Could you check a few things on this model? Use its own coordinates, in mm. Face numbers are marked on the shaded views. A direction names the side the tool comes from. Round coordinates to 2 decimals unless told otherwise and drop trailing zeros. Order: outer loops, then holes, each group sorted by start corner. A loop starts at its lowest first (then second) coordinate and runs counter-clockwise, first axis right, second up. Notation, with made-up numbers: M 75.5,-36.75 L 101.5,-36.75 A31 cw 101.5,-10.75 Z; hole C 25,53 d9. An arc over 180 degrees is marked long. Write each question's results on one line, items separated by ' | '. Start each with the question number.
1. Suppose I cut it at C-C on x = -107. Write out the boundary of the cut face in (y, z), and give its area (3 significant figures).
2. Suppose I cut it at A-A on y = 0. Write out the boundary of the cut face in (x, z), and give its area (3 significant figures).
3. I'm going to push flat-ended pins straight in: pin 1 (1.5 mm diameter, centred on x = -146.5, z = 86, fed in from -Y) (3 decimals); pin 2 (8 mm diameter, centred on y = 8.5, z = 84, fed in from +X); pin 3 (10 mm diameter, centred on y = -5, z = 49.5, fed in from +X). Where does each tip first touch, or does it pass through?
4. For the marked faces 1 and 2, which set-ups out of +Z, -Z, +X, -X, +Y, -Y let a thin tool reach every point of the face, with its end or its side?
5. We'd pull the mould along X, two halves only. Please class the marked faces 3, 4, 5 and 6: released by +X, released by -X, zero draft, split by the parting line, or undercut.
6. Please list where these lines run through material, in increasing order: L1, parallel to Z at x = -109, y = 0; L2, parallel to Y at x = -137, z = 73; L3, parallel to X at y = -29.5, z = 68.
7. Suppose I cut it at B-B on z = 42.5. Write out the boundary of the cut face in (x, y), and give its area (3 significant figures).
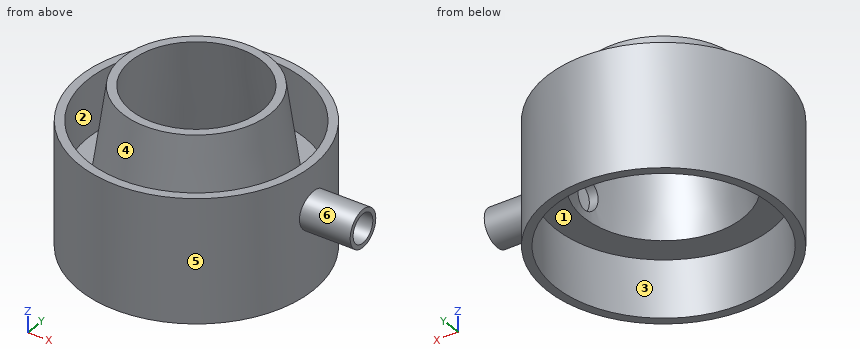
from build123d import *

# Parameters (mm, degrees)
F3_R     = 6.5
F3_R_2   = 5
F4_DEPTH = 20
F5_DEPTH = 14.3


with BuildPart() as f1:
    # F0 (on Front) → F1 (revolve)
    with BuildSketch(Plane.XZ):
        Polygon((-130.0127011951, 91.7292905117), (-133.0127011951, 91.7292905117), (-128.0937719805, 56.7292905117), (-118.0937719805, 56.7292905117), (-118.0937719805, 36.7292905117), (-115.0937719805, 36.7292905117), (-115.0937719805, 79.7292905117), (-118.0937719805, 79.7292905117), (-118.0937719805, 59.7292905117), (-125.5153944847, 59.7292905117), align=None)
    revolve(axis=Axis((-155.8437719805, 0, 54.1304184761), (0, 0, -1)))

    # F3 (on offset) → F4 (join)
    with BuildSketch(Plane.YZ.offset(-118)):
        with Locations((0, 64.2200395022)):
            Circle(F3_R)
        with Locations((0, 64.2200395022)):
            Circle(F3_R_2, mode=Mode.SUBTRACT)
    extrude(amount=F4_DEPTH)

    # F3 (on offset) → F5 (cut, symmetric)
    with BuildSketch(Plane.YZ.offset(-118)):
        with Locations((0, 64.2200395022)):
            Circle(F3_R_2)
    extrude(amount=F5_DEPTH, both=True, mode=Mode.SUBTRACT)


solid = f1.part
Filled sheet:
1) outline: C 0,64.22 d13; hole C 0,64.22 d10 | area: 54.2 mm^2
2) outline: M -196.59,36.73 L -193.59,36.73 L -193.59,56.73 L -183.59,56.73 L -178.67,91.73 L -181.67,91.73 L -186.17,59.73 L -193.59,59.73 L -193.59,79.73 L -196.59,79.73 Z; M -133.01,91.73 L -129.85,69.22 L -126.85,69.22 L -130.01,91.73 Z; M -128.44,59.22 L -128.09,56.73 L -118.09,56.73 L -118.09,36.73 L -115.09,36.73 L -115.09,57.72 L -98,57.72 L -98,59.22 Z; M -118.09,69.22 L -98,69.22 L -98,70.72 L -115.09,70.72 L -115.09,79.73 L -118.09,79.73 Z | area: 499 mm^2
3) pin 1: stops at y = -25.235 | pin 2: stops at x = -129.11 | pin 3: stops at x = -115.09
4) face 1: -Z | face 2: +Z
5) face 3: undercut | face 4: undercut | face 5: split by the parting line | face 6: zero draft
6) L1: z = 57.72 to 59.22, 69.22 to 70.72 | L2: y = -36.13 to -32.71, -21.33 to -17.13, 17.13 to 21.33, 32.71 to 36.13 | L3: x = -183.96 to -179.4, -132.29 to -127.73
7) outline: C -155.84,0 d81.5; hole C -155.84,0 d75.5 | area: 740 mm^2
